Build history of the part. All positions in model axes, mm. A direction names the side the tool comes from. Give positions to 0.01 mm unless a question says otherwise; leave off trailing zeros. Loops run counter-clockwise (first coordinate to the right, second up) from the corner with the lowest first, then second, coordinate; pieces in that order, holes last. Notation, with made-up numbers: (-16.5, -30.75) -> (-0.5, -30.75) arc R16 cw to (-0.5, -16.75) -> close; hole circle Ø2 at (-39.75, 77). An arc over 180 degrees is marked (long way). One line per question, with ' | ' between items. Start each with the question number.
(1) Slice it at C-C, the plane x = -1. Write the cut outline in (y, z), then the cut area to 3 significant figures.
(2) Flat gauge pins, fed straight in: pin 1 Ø1.5 at (x, z) = (1, 15.5) entering from +Y; pin 2 Ø3 at (x, z) = (-1, -6) entering from -Y; pin 3 Ø2 at (x, z) = (1, -8.5) entering from +Y. Where does each tip first touch, or does it go through?
(3) Slice it at A-A, the plane y = 0. Write the cut outline in (x, z), then the cut area to 3 significant figures.
(4) 3-axis set-ups, long thin cutter, end or side, ignore diameter. For faces 5 (the face through (0, 44.5, 0)), 6 (the face through (-4, -108, 0)): which of +Z, -Z, +X, -X, +Y, -Y reach the whole face in a straight line?
(5) Drill centre lines: L1, parallel to Y at x = 0, z = 0; L2, parallel to Y at x = -3, z = 1; L3, parallel to Y at x = 3.75, z = 11. Where is each one in solid material? Low to high. Write a range as from..to.
(6) Mould opens along Z. For faces 1 (the face through (0, 60, 0)), 2 (the face through (-0.056, -268.872, -4.614)), 3 (the face through (0, -108, 20)), 4 (the face through (4, -108, 0)) say: pulls with the +Z half, pulls with the -Z half, needs draft (parallel to the pull), parting line crosses it, or undercut.
(7) Slice it at D-D, the plane y = -150. Write the cut outline in (x, z), then the cut area to 3 significant figures.
(8) Slice it at B-B, the plane z = 0. Write the cut outline in (x, y).
```python
from build123d import *

# Parameters (mm, degrees)
BOSS_EXTRUDE1_DEPTH      = 4
BOSS_EXTRUDE1_DEPTH_BACK = 4
SKETCH2_R                = 14
SKETCH2_R_2              = 10
SKETCH2_W                = 9
SKETCH2_H                = 9


with BuildPart() as part:
    # Sketch2 → Boss-Extrude1 (new, two sides: drawn at the far end of the back side and taken through both)
    with BuildSketch(Plane(origin=(0, 0, 0), x_dir=(0, 0, -1), z_dir=(1, 0, 0)).offset(-BOSS_EXTRUDE1_DEPTH_BACK)):
        with BuildLine():
            Line((-20, 40), (-20, -260))
            ThreePointArc((-20, -260), (0, -280), (20, -260))
            Line((20, -260), (20, 40))
            ThreePointArc((20, 40), (0, 60), (-20, 40))
        make_face()
        Circle(SKETCH2_R, mode=Mode.SUBTRACT)
        with Locations((0, -150)):
            Circle(SKETCH2_R_2, mode=Mode.SUBTRACT)
        with Locations((0, -260)):
            Circle(SKETCH2_R_2, mode=Mode.SUBTRACT)
        with Locations((0, 40)):
            Rectangle(SKETCH2_W, SKETCH2_H, mode=Mode.SUBTRACT)
    extrude(amount=BOSS_EXTRUDE1_DEPTH + BOSS_EXTRUDE1_DEPTH_BACK)


solid = part.part
```
Final values:
1) outline: (-260, -20) -> (40, -20) arc R20 ccw to (40, 20) -> (-260, 20) arc R20 ccw to start; hole circle Ø20 at (-260, 0); hole circle Ø20 at (-150, 0); hole circle Ø28 at (0, 0); hole (35.5, -4.5) -> (44.5, -4.5) -> (44.5, 4.5) -> (35.5, 4.5) -> close | area: 11,900 mm2
2) pin 1: y = 53.51 | pin 2: y = -279.49 | pin 3: y = 58.54
3) outline: (-4, -20) -> (4, -20) -> (4, -14) -> (-4, -14) -> close; (-4, 14) -> (4, 14) -> (4, 20) -> (-4, 20) -> close | area: 96.0 mm2
4) face 5: +X, -X | face 6: +Z, -Z, -X, +Y, -Y
5) L1: -280..-270, -250..-160, -140..-14, 14..35.5, 44.5..60 | L2: -279.97..-269.95, -250.05..-159.95, -140.05..-13.96, 13.96..35.5, 44.5..59.97 | L3: -276.7..-8.66, 8.66..56.7
6) face 1: parting line crosses it | face 2: undercut | face 3: pulls with the +Z half | face 4: needs draft
7) outline: (-4, -20) -> (4, -20) -> (4, -10) -> (-4, -10) -> close; (-4, 10) -> (4, 10) -> (4, 20) -> (-4, 20) -> close | area: 160 mm2
8) outline: (-4, -280) -> (4, -280) -> (4, -270) -> (-4, -270) -> close; (-4, -250) -> (4, -250) -> (4, -160) -> (-4, -160) -> close; (-4, -140) -> (4, -140) -> (4, -14) -> (-4, -14) -> close; (-4, 14) -> (4, 14) -> (4, 35.5) -> (-4, 35.5) -> close; (-4, 44.5) -> (4, 44.5) -> (4, 60) -> (-4, 60) -> close
